The drawing under review shows one solid part. Ordinate dimensions are in mm from its lowest x, y, z. Round coordinates to 2 decimals unless told otherwise and drop trailing zeros. Write each loop counter-clockwise with the first axis right and the second up, starting at its lowest first coordinate (ties: lowest second). Pieces come first, ordered by that corner, then holes. Notation, with made-up numbers: M -34.75,-8.5 L 8.25,-8.5 A26 ccw 8.25,9.5 Z; hole C -4.75,40.5 d5. An arc over 180 degrees is marked long. One line per item, written item: value. Start each with the question number.
1) Take a section at B-B, the plane x = 10. Write out the cut boundary in (y, z), and give its area (3 significant figures).
2) Mouldability with a two-part tool opening along Y and no side actions: class the marked faces 1, 2 and 3 as +Y half, -Y half, draft (parallel to the pull), parting line (faces both ways), or undercut.
3) Wall thickness on probe 1 along Y at (x, z) = (10, 9.5); probe 2 along X at (y, z) = (1.5, 19.25); probe 3 along X at (y, z) = (29.25, 18): over which ranges is each line inside the solid? List them lowest first.
4) Take a section at C-C, the plane z = 2.75. Write out the cut boundary in (x, y), and give its area (3 significant figures).
5) Take a section at D-D, the plane x = 3.25. Write out the cut boundary in (y, z), and give its area (3 significant figures).
6) For P1, Ø2, axis at y = 23.5, z = 11, coming from the -X side, flat-tipped, find the tip position at first contact; note if it passes through.
7) Take a section at A-A, the plane y = 15. Write out the cut boundary in (x, z), and give its area (3 significant figures).
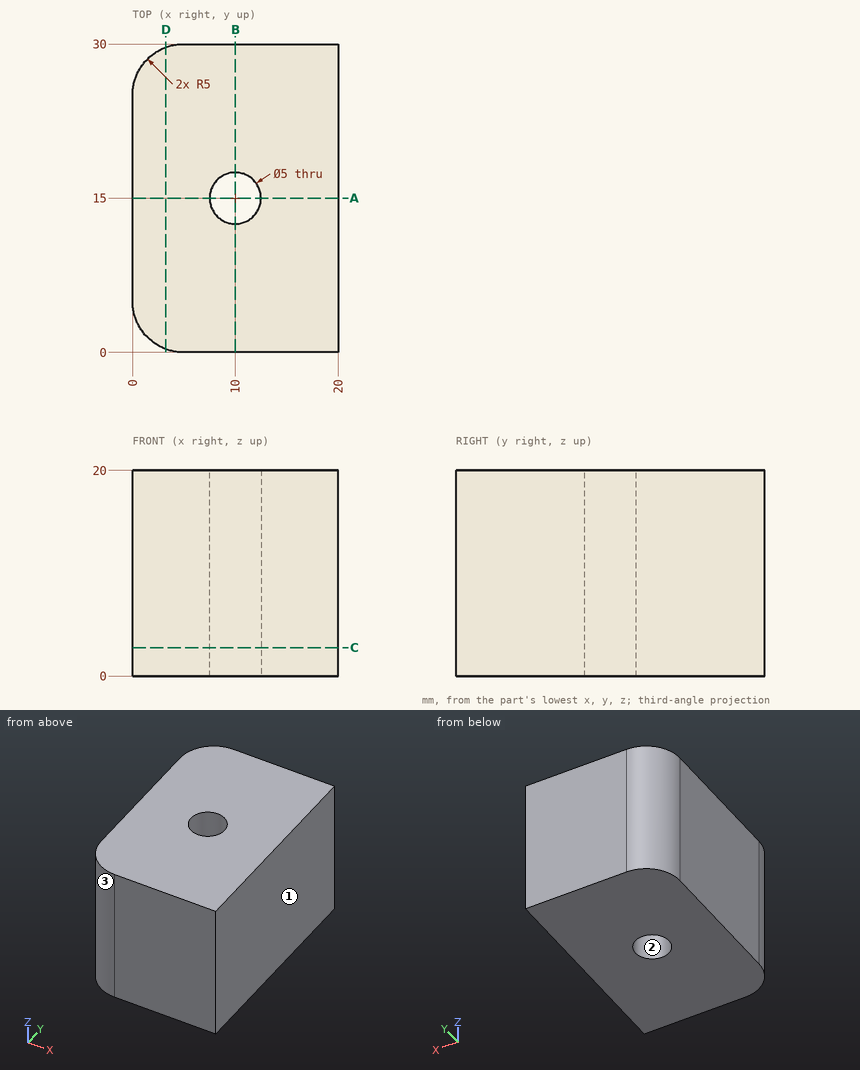
Checked values:
1. outline: M 0,0 L 12.5,0 L 12.5,20 L 0,20 Z; M 17.5,0 L 30,0 L 30,20 L 17.5,20 Z
1. area: 500 mm2
2. face 1: draft
2. face 2: undercut
2. face 3: -Y half
3. probe 1: y = 0 to 12.5, 17.5 to 30
3. probe 2: x = 1.43 to 20
3. probe 3: x = 2.37 to 20
4. outline: M 0,5 A5 ccw 5,0 L 20,0 L 20,30 L 5,30 A5 ccw 0,25 Z; hole C 10,15 d5
4. area: 570 mm2
5. outline: M 0.32,0 L 29.68,0 L 29.68,20 L 0.32,20 Z
5. area: 587 mm2
6. P1: stops at x = 0
7. outline: M 0,0 L 7.5,0 L 7.5,20 L 0,20 Z; M 12.5,0 L 20,0 L 20,20 L 12.5,20 Z
7. area: 300 mm2
